```python
from build123d import *

# Parameters (mm, degrees)
BOSS_EXTRUDE1_DEPTH     = 10.8
BOSS_EXTRUDE2_DEPTH     = 1.8
CUT_EXTRUDE1_DEPTH      = 15.9231364
CUT_EXTRUDE2_DEPTH      = 19.995262567
CUT_EXTRUDE2_DEPTH_BACK = 19.995262567
SKETCH4_W               = 8.1
SKETCH4_H               = 1.7
SKETCH6_R               = 1
BOSS_EXTRUDE3_DEPTH     = 0.8


with BuildPart() as part:
    # Sketch1 → Boss-Extrude1 (new body)
    with BuildSketch(Plane(origin=(0, 0, 0), x_dir=(1, 0, 0), z_dir=(0, 1, 0))):
        Polygon((2.7, -6.3), (4.2, -4.8), (4.2, 6.3), (-4.2, 6.3), (-4.2, -4.8), (-2.7, -6.3), align=None)
    extrude(amount=BOSS_EXTRUDE1_DEPTH)

    # Sketch2 → Boss-Extrude2 (add)
    with BuildSketch(Plane(origin=(0, 10.8, 0), x_dir=(1, 0, 0), z_dir=(0, 1, 0))):
        with BuildLine():
            Line((-7.5, -0.7), (7.5, -0.7))
            ThreePointArc((7.5, -0.7), (9.338477631, 0.061522369), (10.1, 1.9))
            Line((10.1, 1.9), (10.1, 3.7))
            ThreePointArc((10.1, 3.7), (9.338477631, 5.538477631), (7.5, 6.3))
            Line((7.5, 6.3), (-7.5, 6.3))
            ThreePointArc((-7.5, 6.3), (-9.338477631, 5.538477631), (-10.1, 3.7))
            Line((-10.1, 3.7), (-10.1, 1.9))
            ThreePointArc((-10.1, 1.9), (-9.338477631, 0.061522369), (-7.5, -0.7))
        make_face()
    extrude(amount=-BOSS_EXTRUDE2_DEPTH)

    # Sketch3 → Cut-Extrude1 (cut, through all)
    with BuildSketch(Plane.XZ.offset(-9)):
        with BuildLine():
            Line((6.1, -4), (6.1, -2.6))
            ThreePointArc((6.1, -2.6), (7.5, -1.2), (8.9, -2.6))
            Line((8.9, -2.6), (8.9, -4))
            ThreePointArc((8.9, -4), (7.5, -5.4), (6.1, -4))
        make_face()
        with BuildLine():
            Line((-6.1, -4), (-6.1, -2.6))
            ThreePointArc((-6.1, -2.6), (-7.5, -1.2), (-8.9, -2.6))
            Line((-8.9, -2.6), (-8.9, -4))
            ThreePointArc((-8.9, -4), (-7.5, -5.4), (-6.1, -4))
        make_face()
    extrude(amount=-CUT_EXTRUDE1_DEPTH, mode=Mode.SUBTRACT)

    # Sketch4 → Cut-Extrude2 (cut, two sides: drawn at the far end of the back side and taken through both)
    with BuildSketch(Plane(origin=(4.2, 0, 0), x_dir=(0, 0, -1), z_dir=(1, 0, 0)).offset(-CUT_EXTRUDE2_DEPTH_BACK)):
        with Locations((-2.25, 6.05)):
            Rectangle(SKETCH4_W, SKETCH4_H)
    extrude(amount=CUT_EXTRUDE2_DEPTH + CUT_EXTRUDE2_DEPTH_BACK, mode=Mode.SUBTRACT)

    # Sketch6 → Boss-Extrude3 (add)
    with BuildSketch(Plane(origin=(0, 10.8, 0), x_dir=(1, 0, 0), z_dir=(0, 1, 0))):
        with Locations(Location((0, -2.4, 0), (0, 0, 90))):
            Circle(SKETCH6_R)
        with Locations(Location((0, 4, 0), (0, 0, 90))):
            Circle(SKETCH6_R)
    extrude(amount=BOSS_EXTRUDE3_DEPTH)


solid = part.part
```
Check sheet for the modelled part. Datum: model origin and axes. Units: mm. A direction names the side the tool comes from. Give positions to 0.01 mm unless a question says otherwise; leave off trailing zeros. Write each loop counter-clockwise with the first axis right and the second up, starting at its lowest first coordinate (ties: lowest second). Pieces come first, ordered by that corner, then holes.
Item 1: Cross-section at C-C (z = -1.5). Enter the section's corners in (x, y), and give its area (3 significant figures).
Item 2: Access from +Z, -Z, +X, -X, +Y, -Y to the whole of each face (thin tool, end or side, straight path). Record for faces 1 (the face through (0, 6, -1.8)), 2 (the face through (-8.9, 10, -3)), 3 (the face through (6, 10, 0.7)).
Item 3: Scan lines: L1, parallel to Y at x = 1.75, z = -0.75; L2, parallel to X at y = 10.25, z = -1.75; L3, parallel to Y at x = 0.25, z = 1.75. Record each from-to range of solid material in increasing order.
Item 4: Draft check along Z on faces 4 (the face through (-7.5, 9.9, -1.2)), 5 (the face through (0, 7, -6.3)), 6 (the face through (0, 9, 6.3)), 7 (the face through (10.1, 10, -3)). Enter one of: released by +Z, released by -Z, zero draft, split by the parting line, or undercut.
Item 5: Cross-section at D-D (y = 1). Enter the section's corners in (x, z).
Item 6: Cross-section at A-A (z = 2.4). Enter the section's corners in (x, y).
Item 7: Gauge pin test, flat ends, axial feed: pin 1 (2 mm diameter, centred on x = 5, y = 10, fed in from +Z); pin 2 (3 mm diameter, centred on y = 6, z = 0.5, fed in from -X); pin 3 (4.5 mm diameter, centred on x = -7.5, z = -3.5, fed in from -Y). Record the tip position at first contact, or that the pin passes through.
Item 8: Cross-section at B-B (x = 0). Enter the section's corners in (y, z).
Report:
1. outline: (-10.07, 9) - (-8.37, 9) - (-8.37, 10.8) - (-10.07, 10.8) - close; (-6.63, 9) - (-4.2, 9) - (-4.2, 6.9) - (4.2, 6.9) - (4.2, 9) - (6.63, 9) - (6.63, 10.8) - (-6.63, 10.8) - close; (-4.2, 0) - (4.2, 0) - (4.2, 5.2) - (-4.2, 5.2) - close; (8.37, 9) - (10.07, 9) - (10.07, 10.8) - (8.37, 10.8) - close
1. area: 91.3 mm2
2. face 1: +Z, +X, -X
2. face 2: +Y, -Y
2. face 3: +Z, +X, +Y, -Y
3. L1: y = 0 to 5.2, 6.9 to 10.8
3. L2: x = -10.1 to -8.61, -6.39 to 6.39, 8.61 to 10.1
3. L3: y = 0 to 5.2, 6.9 to 11.6
4. face 4: undercut
4. face 5: released by -Z
4. face 6: released by +Z
4. face 7: zero draft
5. outline: (-4.2, -6.3) - (4.2, -6.3) - (4.2, 4.8) - (2.7, 6.3) - (-2.7, 6.3) - (-4.2, 4.8) - close
6. outline: (-4.2, 0) - (4.2, 0) - (4.2, 5.2) - (-4.2, 5.2) - close; (-4.2, 6.9) - (4.2, 6.9) - (4.2, 10.8) - (1, 10.8) - (1, 11.6) - (-1, 11.6) - (-1, 10.8) - (-4.2, 10.8) - close
7. pin 1: stops at z = 5
7. pin 2: stops at x = -4.2
7. pin 3: stops at y = 9
8. outline: (0, -6.3) - (10.8, -6.3) - (10.8, -5) - (11.6, -5) - (11.6, -3) - (10.8, -3) - (10.8, 1.4) - (11.6, 1.4) - (11.6, 3.4) - (10.8, 3.4) - (10.8, 6.3) - (6.9, 6.3) - (6.9, -1.8) - (5.2, -1.8) - (5.2, 6.3) - (0, 6.3) - close
